```python
from build123d import *

# Parameters (mm, degrees)
SKETCH_1_W          = 31.2
SKETCH_1_H          = 25
EXTRUDE_1_DEPTH     = 7.1
CUT_EXTRUDE_1_DEPTH = 50.9
SKETCH_3_R          = 1.5
CUT_EXTRUDE_9_DEPTH = 2


with BuildPart() as part:
    # 草图1 → 凸台-拉伸1 (new body)
    with BuildSketch(Plane(origin=(0, 0, 0), x_dir=(1, 0, 0), z_dir=(0, 1, 0))):
        with Locations((15.6, 12.5)):
            Rectangle(SKETCH_1_W, SKETCH_1_H)
    extrude(amount=EXTRUDE_1_DEPTH)

    # 草图2 → 切除-拉伸1 (cut)
    with BuildSketch(Plane.ZY):
        Polygon((-19.5, 0), (-19.5, 1), (-16.5, 1), (-16.5, 2), (-19.5, 2), (-19.5, 3.3), (-12.5, 3.3), (-5.5, 3.3), (-5.5, 2), (-8.5, 2), (-8.5, 1), (-5.5, 1), (-5.5, 0), align=None)
    extrude(amount=-CUT_EXTRUDE_1_DEPTH, mode=Mode.SUBTRACT)

    # 草图3 → 切除-拉伸9 (cut)
    with BuildSketch(Plane(origin=(0, 7.1, 0), x_dir=(1, 0, 0), z_dir=(0, 1, 0))):
        with Locations((10.6, 22)):
            Circle(SKETCH_3_R)
        with Locations((20.6, 22)):
            Circle(SKETCH_3_R)
        with Locations((20.6, 3)):
            Circle(SKETCH_3_R)
        with Locations((10.6, 3)):
            Circle(SKETCH_3_R)
    extrude(amount=-CUT_EXTRUDE_9_DEPTH, mode=Mode.SUBTRACT)


solid = part.part
```
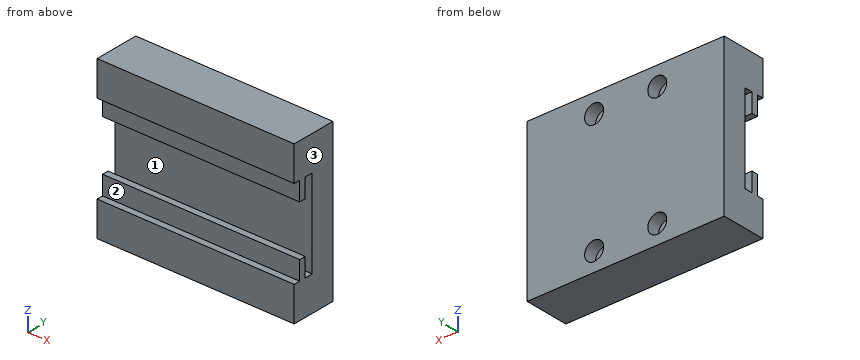
Verification items for the finished model (mm, model axes). Face numbers are marked on the shaded views. Coordinates: 2 decimals unless noted, no trailing zeros. Loops run counter-clockwise (first coordinate to the right, second up) from the corner with the lowest first, then second, coordinate; pieces in that order, holes last. Notation, with made-up numbers: (82, 15.25) -> (100, 15.25) arc R34 cw to (100, 49.25) -> close; hole circle Ø3 at (51, 28). An arc over 180 degrees is marked (long way). Answer in a Markdown table with one row per item. Add a question column.
1. Section check B-B, the plane z = -6.25. Enter the section's corners in (x, y).
2. Section check D-D, the plane x = 10.6. Enter the section's corners in (y, z).
3. Draft check along Y on the marked faces 1, 2 and 3. Enter one of: +Y half, -Y half, draft (parallel to the pull), parting line (faces both ways), or undercut.
4. Material ranges on probe 1 along X at (y, z) = (5.7, -22); probe 2 along Z at (x, y) = (10.6, 5.95); probe 3 along Z at (x, y) = (13, 2.5), recorded low to high. Write a range as [from, to].
5. Section check A-A, the plane y = 1.5. Enter the section's corners in (x, z), then the cut area to 3 significant figures.
6. Depth check by flat-ended pin: P1, Ø3.5, axis at x = 10.6, z = -22, coming from the -Y side; P2, Ø2.5, axis at x = 10, z = -17.5, coming from the -Y side; P3, Ø1.8, axis at x = 20.6, z = -3, coming from the +Y side. Enter the tip coordinate at first touch or a pass-through.
7. Section check C-C, the plane y = 6. Enter the section's corners in (x, z).
Derived:
| question | item | result |
|---|---|---|
| 1 | outline | (0, 1) -> (31.2, 1) -> (31.2, 2) -> (0, 2) -> close; (0, 3.3) -> (31.2, 3.3) -> (31.2, 7.1) -> (0, 7.1) -> close |
| 2 | outline | (0, -25) -> (7.1, -25) -> (7.1, -23.5) -> (5.1, -23.5) -> (5.1, -20.5) -> (7.1, -20.5) -> (7.1, -4.5) -> (5.1, -4.5) -> (5.1, -1.5) -> (7.1, -1.5) -> (7.1, 0) -> (0, 0) -> (0, -5.5) -> (1, -5.5) -> (1, -8.5) -> (2, -8.5) -> (2, -5.5) -> (3.3, -5.5) -> (3.3, -19.5) -> (2, -19.5) -> (2, -16.5) -> (1, -16.5) -> (1, -19.5) -> (0, -19.5) -> close |
| 3 | face 1 | undercut |
| 3 | face 2 | -Y half |
| 3 | face 3 | draft |
| 4 | probe 1 | x = [0, 9.1], [12.1, 19.1], [22.1, 31.2] |
| 4 | probe 2 | z = [-25, -23.5], [-20.5, -4.5], [-1.5, 0] |
| 4 | probe 3 | z = [-25, -19.5], [-5.5, 0] |
| 5 | outline | (0, -25) -> (31.2, -25) -> (31.2, -16.5) -> (0, -16.5) -> close; (0, -8.5) -> (31.2, -8.5) -> (31.2, 0) -> (0, 0) -> close |
| 5 | area | 530 mm² |
| 6 | P1 | stops at y = 0 |
| 6 | P2 | stops at y = 1 |
| 6 | P3 | stops at y = 5.1 |
| 7 | outline | (0, -25) -> (31.2, -25) -> (31.2, 0) -> (0, 0) -> close; hole circle Ø3 at (10.6, -22); hole circle Ø3 at (10.6, -3); hole circle Ø3 at (20.6, -22); hole circle Ø3 at (20.6, -3) |
